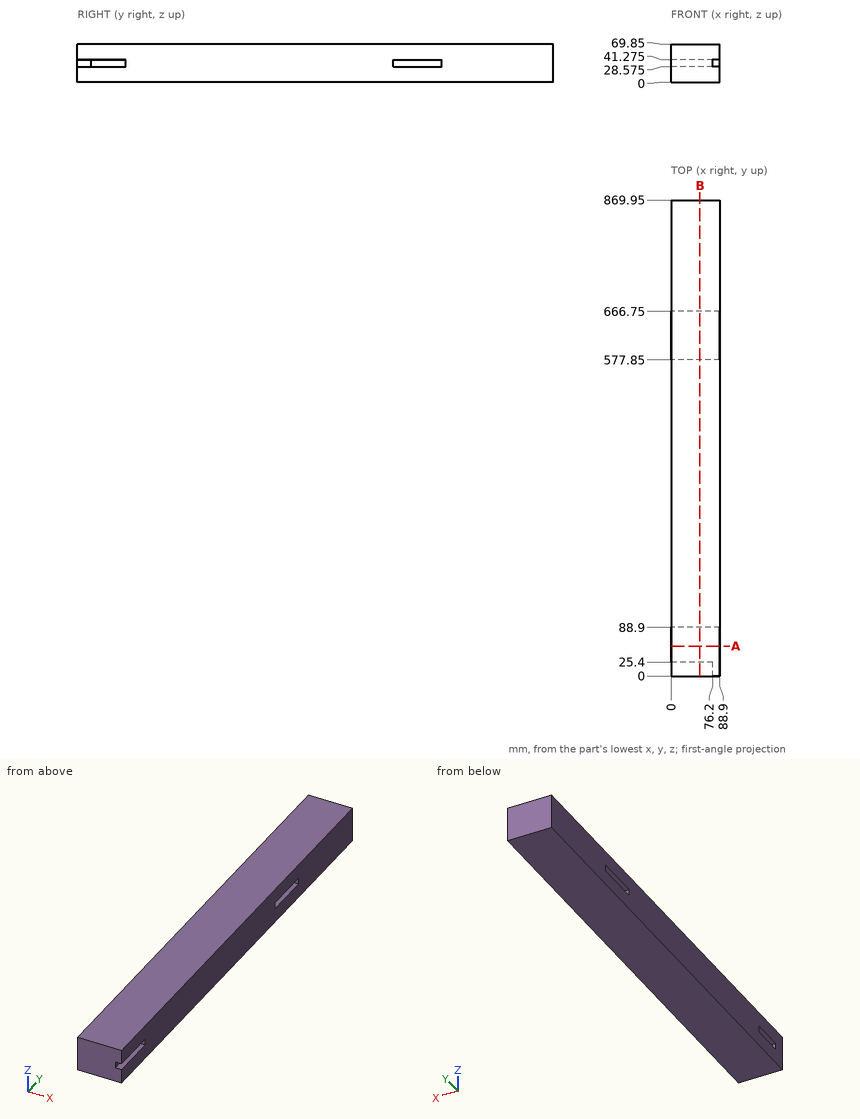
Here's the drawing with two shaded views (mm, measured from the low corner). I have some questions. Give positions to 0.01 mm unless a question says otherwise; leave off trailing zeros. Write each loop counter-clockwise with the first axis right and the second up, starting at its lowest first coordinate (ties: lowest second). Pieces come first, ordered by that corner, then holes. Notation, with made-up numbers: (63, 64.5) - (86, 64.5) arc R12 cw to (86, 87.5) - close; hole circle Ø6 at (20.25, 6.25). An arc over 180 degrees is marked (long way). One line per item, written item: value. Start each with the question number.
Item 1: Please list where these lines run through material, in increasing order: line 1 (Y direction, x = 61.5, z = 37.5); line 2 (Y direction, x = 82.5, z = 34). Write a range as from..to.
Item 2: I'm going to push a flat-ended pin straight in: pin 1 (6.5 mm diameter, centred on y = 9.5, z = 36.5, fed in from +X). Where does the tip first touch, or does it pass through?
Item 3: Imagine slicing it at A-A, the plane y = 54.5. List the corners of the cut face in (x, z) for me (3 decimals).
Item 4: Imagine slicing it at B-B, the plane x = 52.5. List the corners of the cut face in (y, z) for me (3 decimals).
Geometry says:
1. line 1: 0..25.4, 88.9..577.85, 666.75..869.95
1. line 2: 88.9..577.85, 666.75..869.95
2. pin 1: x = 76.2
3. outline: (0, 0) - (88.9, 0) - (88.9, 28.575) - (0, 28.575) - close; (0, 41.275) - (88.9, 41.275) - (88.9, 69.85) - (0, 69.85) - close
4. outline: (0, 0) - (869.95, 0) - (869.95, 69.85) - (0, 69.85) - close; hole (25.4, 28.575) - (88.9, 28.575) - (88.9, 41.275) - (25.4, 41.275) - close; hole (577.85, 28.575) - (666.75, 28.575) - (666.75, 41.275) - (577.85, 41.275) - close
